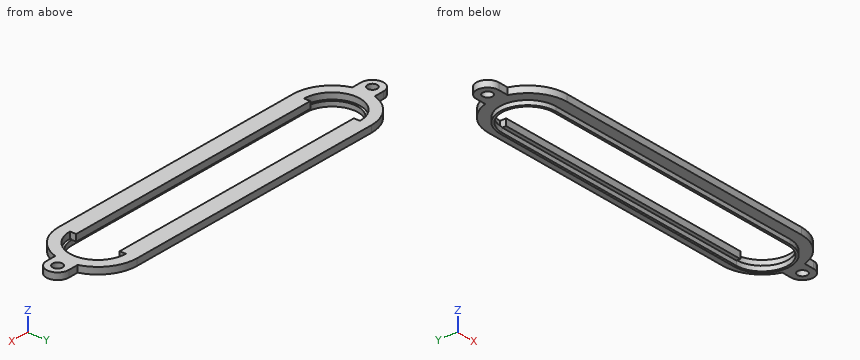
```python
from build123d import *

# Parameters (mm, degrees)
BOSS_EXTRUDE5_DEPTH       = 3.81
SKETCH2_W                 = 158.75
SKETCH2_H                 = 1.27
BOSS_EXTRUDE14_DEPTH      = 2.54
BOSS_EXTRUDE14_DEPTH_BACK = 0.254
SKETCH3_R                 = 2.794
SKETCH3_R_2               = 2.820459539
BOSS_EXTRUDE15_DEPTH      = 3.81


with BuildPart() as part:
    # Sketch1 → Boss-Extrude5 (new body)
    with BuildSketch(Plane.XY):
        with BuildLine():
            Line((19.130596058, -22.225), (177.880596058, -22.225))
            ThreePointArc((177.880596058, -22.225), (200.105596058, 0), (177.880596058, 22.225))
            Line((177.880596058, 22.225), (19.130596058, 22.225))
            ThreePointArc((19.130596058, 22.225), (-3.094403942, 0), (19.130596058, -22.225))
        make_face()
        with BuildLine():
            Line((19.130596058, -12.319), (19.130596058, -15.875))
            ThreePointArc((19.130596058, -15.875), (3.255596058, 0), (19.130596058, 15.875))
            Line((19.130596058, 15.875), (19.130596058, 12.319))
            Line((19.130596058, 12.319), (177.880596058, 12.319))
            Line((177.880596058, 12.319), (177.880596058, 15.875))
            ThreePointArc((177.880596058, 15.875), (193.755596058, 0), (177.880596058, -15.875))
            Line((177.880596058, -15.875), (177.880596058, -12.319))
            Line((177.880596058, -12.319), (19.130596058, -12.319))
        make_face(mode=Mode.SUBTRACT)
    extrude(amount=BOSS_EXTRUDE5_DEPTH)

    # Sketch2 → Boss-Extrude14 (add, two sides)
    with BuildSketch(Plane(origin=(0, 0, 0), x_dir=(-1, 0, 0), z_dir=(0, 0, -1))) as boss_extrude14_sk:
        with BuildLine():
            ThreePointArc((-177.880596058, -14.605), (-192.485596058, 0), (-177.880596058, 14.605))
            Line((-177.880596058, 14.605), (-177.880596058, 15.875))
            ThreePointArc((-177.880596058, 15.875), (-193.755596058, 0), (-177.880596058, -15.875))
            Line((-177.880596058, -15.875), (-177.880596058, -14.605))
        make_face()
        Polygon((-177.880596058, 15.875), (-177.880596058, 14.605), (-19.130596058, 14.605), (-19.130596058, 14.665246221), (-19.130596058, 15.875), align=None)
        with Locations((-98.505596058, -15.24)):
            Rectangle(SKETCH2_W, SKETCH2_H)
        with BuildLine():
            Line((-19.130596058, 14.665246221), (-19.130596058, 14.605))
            ThreePointArc((-19.130596058, 14.605), (-4.525596058, 0), (-19.130596058, -14.605))
            Line((-19.130596058, -14.605), (-19.130596058, -15.875))
            ThreePointArc((-19.130596058, -15.875), (-3.255596058, 0), (-19.130596058, 15.875))
            Line((-19.130596058, 15.875), (-19.130596058, 14.665246221))
        make_face()
    extrude(amount=BOSS_EXTRUDE14_DEPTH)
    extrude(boss_extrude14_sk.sketch, amount=-BOSS_EXTRUDE14_DEPTH_BACK)

    # Sketch3 → Boss-Extrude15 (add)
    with BuildSketch(Plane.XY.offset(3.81)):
        with BuildLine():
            Line((-8.174403942, 6.35), (-2.167951427, 6.35))
            ThreePointArc((-2.167951427, 6.35), (-3.094403942, 0), (-2.167951427, -6.35))
            Line((-2.167951427, -6.35), (-8.174403942, -6.35))
            ThreePointArc((-8.174403942, -6.35), (-14.524403942, 0), (-8.174403942, 6.35))
        make_face()
        with Locations((-8.174403942, 0)):
            Circle(SKETCH3_R, mode=Mode.SUBTRACT)
        with BuildLine():
            Line((205.185596058, -6.35), (199.179143544, -6.35))
            ThreePointArc((199.179143544, -6.35), (200.105596058, 0), (199.179143544, 6.35))
            Line((199.179143544, 6.35), (205.185596058, 6.35))
            ThreePointArc((205.185596058, 6.35), (211.535596058, 0), (205.185596058, -6.35))
        make_face()
        with Locations((205.185596058, 0)):
            Circle(SKETCH3_R_2, mode=Mode.SUBTRACT)
    extrude(amount=-BOSS_EXTRUDE15_DEPTH)


solid = part.part
```
Source: CAD feature listing. Evaluate the final solid. Frame: model axes, mm. Give positions to 0.01 mm unless a question says otherwise; leave off trailing zeros. Write each loop counter-clockwise with the first axis right and the second up, starting at its lowest first coordinate (ties: lowest second). Pieces come first, ordered by that corner, then holes.
1. First-contact query: pin 1 (1.3 mm diameter, centred on x = 88.5, z = -1, fed in from +Y) (3 decimals); pin 2 (0.8 mm diameter, centred on x = 87.5, z = -1.5, fed in from -Y) (3 decimals); pin 3 (1 mm diameter, centred on y = 5.5, z = 2.5, fed in from +X). Flat tips, straight axial feed; report the tip coordinate or a pass-through.
2. Section query D-D (y = -9). Return the cut outline in (x, z).
3. Section query C-C (x = 142). Return the cut outline in (y, z) (3 decimals), then the cut area to 3 significant figures.
4. Material intervals for line 1 along Y through (x, z) = (110.5, -0.25) (3 decimals); line 2 along Y through (x, z) = (53, 2.75) (3 decimals); line 3 along X through (y, z) = (2.5, 2.25), sorted ascending.
5. Section query A-A (y = 0). Return the cut outline in (x, z).
6. Section query B-B (z = 2.25). Return the cut outline in (x, y) (3 decimals).
Output values:
1. pin 1: stops at y = 15.875
1. pin 2: stops at y = -15.875
1. pin 3: stops at x = 209.1
2. outline: (-1.19, 0) - (6.05, 0) - (6.05, -2.54) - (7.63, -2.54) - (7.63, 0.25) - (6.05, 0.25) - (6.05, 3.81) - (-1.19, 3.81) - close; (189.38, -2.54) - (190.96, -2.54) - (190.96, 0) - (198.2, 0) - (198.2, 3.81) - (190.96, 3.81) - (190.96, 0.25) - (189.38, 0.25) - close
3. outline: (-22.225, 0) - (-15.875, 0) - (-15.875, -2.54) - (-14.605, -2.54) - (-14.605, 0) - (-12.319, 0) - (-12.319, 3.81) - (-22.225, 3.81) - close; (12.319, 0) - (14.605, 0) - (14.605, -2.54) - (15.875, -2.54) - (15.875, 0) - (22.225, 0) - (22.225, 3.81) - (12.319, 3.81) - close
3. area: 81.9 mm2
4. line 1: y = -15.875 to -14.605, 14.605 to 15.875
4. line 2: y = -22.225 to -12.319, 12.319 to 22.225
4. line 3: x = -14.01 to -9.42, -6.93 to 3.45, 193.56 to 203.88, 206.49 to 211.02
5. outline: (-14.52, 0) - (-10.97, 0) - (-10.97, 3.81) - (-14.52, 3.81) - close; (-5.38, 0) - (3.26, 0) - (3.26, -2.54) - (4.53, -2.54) - (4.53, 0.25) - (3.26, 0.25) - (3.26, 3.81) - (-5.38, 3.81) - close; (192.49, -2.54) - (193.76, -2.54) - (193.76, 0) - (202.37, 0) - (202.37, 3.81) - (193.76, 3.81) - (193.76, 0.25) - (192.49, 0.25) - close; (208.01, 0) - (211.54, 0) - (211.54, 3.81) - (208.01, 3.81) - close
6. outline: (-8.174, -6.35) - (-2.168, -6.35) arc R22.225 ccw to (19.131, -22.225) - (177.881, -22.225) arc R22.225 ccw to (199.179, -6.35) - (205.186, -6.35) arc R6.35 ccw to (205.186, 6.35) - (199.179, 6.35) arc R22.225 ccw to (177.881, 22.225) - (19.131, 22.225) arc R22.225 ccw to (-2.168, 6.35) - (-8.174, 6.35) arc R6.35 ccw to start; hole circle Ø5.588 at (-8.174, 0); hole (19.131, -15.875) - (19.131, -12.319) - (177.881, -12.319) - (177.881, -15.875) arc R15.875 ccw to (177.881, 15.875) - (177.881, 12.319) - (19.131, 12.319) - (19.131, 15.875) arc R15.875 ccw to start; hole circle Ø5.641 at (205.186, 0)
